```python
from build123d import *

# Parameters (mm, degrees)
SKETCH1_R           = 5.25
BOSS_EXTRUDE1_DEPTH = 100
BOSS_EXTRUDE2_DEPTH = 2.5
SKETCH3_OUTSIDE_W   = 35.74
SKETCH3_OUTSIDE_H   = 35.74
SKETCH3_OUTSIDE_R   = 5.25
CUT_EXTRUDE1_DEPTH  = 101.275246198
SKETCH4_R           = 4
CUT_EXTRUDE2_DEPTH  = 116.629526938
SKETCH5_R           = 2.65
CUT_EXTRUDE3_DEPTH  = 6


with BuildPart() as part:
    # Sketch1 → Boss-Extrude1 (new body)
    with BuildSketch(Plane(origin=(0, 0, 0), x_dir=(1, 0, 0), z_dir=(0, 1, 0))):
        with Locations(Location((0, 0, 0), (0, 0, 270))):
            Circle(SKETCH1_R)
    extrude(amount=BOSS_EXTRUDE1_DEPTH)

    # Sketch2 → Boss-Extrude2 (add, symmetric)
    with BuildSketch(Plane.XY):
        with BuildLine():
            Line((-5.25, 100), (-5.25, 110))
            ThreePointArc((-5.25, 110), (0, 115.25), (5.25, 110))
            Line((5.25, 110), (5.25, 100))
            Line((5.25, 100), (-5.25, 100))
        make_face()
    extrude(amount=BOSS_EXTRUDE2_DEPTH, both=True)

    # Sketch3 outside → Cut-Extrude1 (cut, through all)
    with BuildSketch(Plane(origin=(0, 100, 0), x_dir=(1, 0, 0), z_dir=(0, 1, 0))):
        Rectangle(SKETCH3_OUTSIDE_W, SKETCH3_OUTSIDE_H)
        with Locations(Location((0, 0, 0), (0, 0, 151.563109851))):
            Circle(SKETCH3_OUTSIDE_R, mode=Mode.SUBTRACT)
    extrude(amount=CUT_EXTRUDE1_DEPTH, mode=Mode.SUBTRACT)

    # Sketch4 → Cut-Extrude2 (cut, through all)
    with BuildSketch(Plane.XY.offset(2.5)):
        with Locations((0, 110)):
            Circle(SKETCH4_R)
    extrude(amount=-CUT_EXTRUDE2_DEPTH, mode=Mode.SUBTRACT)

    # Sketch5 → Cut-Extrude3 (cut)
    with BuildSketch(Plane.XZ):
        with Locations(Location((0, 0, 0), (0, 0, 270))):
            Circle(SKETCH5_R)
    extrude(amount=-CUT_EXTRUDE3_DEPTH, mode=Mode.SUBTRACT)


solid = part.part
```
For this review, take the finished solid that the model builds, in its own axes (mm). A direction names the side the tool comes from. Give positions to 0.01 mm unless a question says otherwise; leave off trailing zeros. Write each loop counter-clockwise with the first axis right and the second up, starting at its lowest first coordinate (ties: lowest second). Pieces come first, ordered by that corner, then holes.
Item 1: The part is to be moulded in two halves that separate along Z. For faces 4 (the face through (0, 104, -2.5)), 5 (the face through (-0.521, 113.966, 0.035)), 6 (the face through (0, 6, 0)), say which applies: +Z half, -Z half, draft (parallel to the pull), parting line (faces both ways), or undercut.
Item 2: Insertion check: P1, Ø6, axis at x = 0.5, z = 1, coming from the -Y side; P2, Ø0.8, axis at x = -1.5, z = -4, coming from the +Y side; P3, Ø1, axis at y = 83, z = 2, coming from the +X side; P4, Ø3, axis at x = 0, z = 0, coming from the -Y side. Each pin has a flat end and moves straight along its axis. Give the tip position at first contact, or say it passes through.
Item 3: Machinability: for faces 1 (the face through (-1.612, 2.958, 2.103)), 2 (the face through (0, 104, 2.5)), 3 (the face through (0, 100, -4)), which of the approach directions +Z, -Z, +X, -X, +Y, -Y give a long, thin tool a straight path to every point of the face, cutting with its end or side? Answer none if there is none.
Item 4: Take a section at A-A (x = 0). Give the boundary of the cut face in (y, z).
Item 5: Take a section at D-D (z = -4.25). Give the boundary of the cut face in (x, y), and give its area (3 significant figures).
Item 6: Take a section at C-C (y = 20). Give the boundary of the cut face in (x, z), and give its area (3 significant figures).
Item 7: Take a section at B-B (z = 0). Give the boundary of the cut face in (x, y).
Item 8: Wall thickness on probe 1 along X at (y, z) = (3.9, 0); probe 2 along Y at (x, z) = (2.5, 0); probe 3 along Z at (x, y) = (0.25, 32.5): over which ranges is each line inside the solid? List them lowest first.
Established:
1. face 4: -Z half
1. face 5: draft
1. face 6: undercut
2. P1: stops at y = 0
2. P2: stops at y = 100
2. P3: stops at x = 5.03
2. P4: stops at y = 6
3. face 1: -Y
3. face 2: +Z, +X, -X, +Y
3. face 3: -Z, +X, -X, +Y
4. outline: (0, -5.25) - (100, -5.25) - (100, -2.5) - (106, -2.5) - (106, 2.5) - (100, 2.5) - (100, 5.25) - (0, 5.25) - (0, 2.65) - (6, 2.65) - (6, -2.65) - (0, -2.65) - close; (114, -2.5) - (115.25, -2.5) - (115.25, 2.5) - (114, 2.5) - close
5. outline: (-3.08, 0) - (3.08, 0) - (3.08, 100) - (-3.08, 100) - close
5. area: 616 mm2
6. outline: circle Ø10.5 at (0, 0)
6. area: 86.6 mm2
7. outline: (-5.25, 0) - (-2.65, 0) - (-2.65, 6) - (2.65, 6) - (2.65, 0) - (5.25, 0) - (5.25, 110) arc R5.25 ccw to (-5.25, 110) - close; hole circle Ø8 at (0, 110)
8. probe 1: x = -5.25 to -2.65, 2.65 to 5.25
8. probe 2: y = 6 to 106.88, 113.12 to 114.62
8. probe 3: z = -5.24 to 5.24
